```python
from build123d import *

# Parameters (mm, degrees)
SKETCH_1_W       = 100
SKETCH_1_H       = 50
EXTRUDE_1_DEPTH  = 10
F_10_0MM_1_D     = 10
F_10_0MM_1_DEPTH = 23.75
F_10_0MM_1_TIP   = 3.004303095
M10X1_25_1_D     = 8.8
M10X1_25_1_DEPTH = 23.75
M10X1_25_1_TIP   = 2.643786724
FILLET_1_R       = 1
CHAMFER_1_SIZE   = 1
CHAMFER_2_SIZE   = 0.5
FILLET_2_R       = 1


with BuildPart() as part:
    # 草圖1 → 填料-伸長1 (new body)
    with BuildSketch(Plane(origin=(0, 0, 0), x_dir=(1, 0, 0), z_dir=(0, 1, 0))):
        with Locations((50, 25)):
            Rectangle(SKETCH_1_W, SKETCH_1_H)
    extrude(amount=EXTRUDE_1_DEPTH)

    # Ø10.0mm 定位孔1
    with Locations(Plane(origin=(80, 10, -37.5), x_dir=(0, 0, 1), z_dir=(0, 1, 0))):
        with Locations((0, 0), (25, 0)):
            Hole(F_10_0MM_1_D / 2, depth=F_10_0MM_1_DEPTH)
            with Locations((0, 0, -(F_10_0MM_1_DEPTH + F_10_0MM_1_TIP / 2))):  # 118° drill point
                Cone(0, F_10_0MM_1_D / 2, F_10_0MM_1_TIP, mode=Mode.SUBTRACT)

    # M10x1.25 螺紋孔1
    with Locations(Plane(origin=(20, 10, -37.5), x_dir=(0, 0, 1), z_dir=(0, 1, 0))):
        with Locations((0, 0), (25, 0)):
            Hole(M10X1_25_1_D / 2, depth=M10X1_25_1_DEPTH)
            with Locations((0, 0, -(M10X1_25_1_DEPTH + M10X1_25_1_TIP / 2))):  # 118° drill point
                Cone(0, M10X1_25_1_D / 2, M10X1_25_1_TIP, mode=Mode.SUBTRACT)

    # 圓角1
    fillet_1_edges = [part.edges().sort_by_distance(p)[0] for p in [
        (0, 5, -50),
        (100, 5, -50),
        (100, 5, 0),
        (0, 5, 0),
    ]]
    fillet(fillet_1_edges, radius=FILLET_1_R)

    # 導角1
    chamfer_1_edges = [part.edges().sort_by_distance(p)[0] for p in [
        (50, 0, -50),
        (0, 0, -25),
        (100, 0, -25),
        (50, 0, 0),
        (99.707106781, 0, -0.292893219),
        (0.292893219, 0, -0.292893219),
        (0.292893219, 0, -49.707106781),
        (99.707106781, 0, -49.707106781),
    ]]
    chamfer(chamfer_1_edges, length=CHAMFER_1_SIZE)

    # 導角2
    chamfer_2_edges = [part.edges().sort_by_distance(p)[0] for p in [
        (80, 10, -7.5),
        (80, 10, -32.5),
    ]]
    chamfer(chamfer_2_edges, length=CHAMFER_2_SIZE)

    # 圓角2
    fillet_2_edges = [part.edges().sort_by_distance(p)[0] for p in [
        (50, 10, -50),
        (100, 10, -25),
        (0, 10, -25),
        (50, 10, 0),
        (99.707106781, 10, -0.292893219),
        (0.292893219, 10, -0.292893219),
        (0.292893219, 10, -49.707106781),
        (99.707106781, 10, -49.707106781),
    ]]
    fillet(fillet_2_edges, radius=FILLET_2_R)


solid = part.part
```
Check sheet for the modelled part. Datum: model origin and axes. Units: mm. Give positions to 0.01 mm unless a question says otherwise; leave off trailing zeros. Write each loop counter-clockwise with the first axis right and the second up, starting at its lowest first coordinate (ties: lowest second). Pieces come first, ordered by that corner, then holes.
Item 1: Cross-section at A-A (x = 20). Enter the section's corners in (y, z), and give its area (3 significant figures).
Item 2: Cross-section at B-B (z = -37.5). Enter the section's corners in (x, y).
Item 3: Draft check along X on faces 1 (the face through (21.322, 4.93, -41.697)), 2 (the face through (100, 5, -25)), 3 (the face through (49, 5, -50)), 4 (the face through (75.12, 4.68, -11.42)). Enter one of: released by +X, released by -X, zero draft, split by the parting line, or undercut.
Item 4: Cross-section at D-D (x = 80). Enter the section's corners in (y, z).
Item 5: Scan lines: L1, parallel to X at y = 2.25, z = -12.5; L2, parallel to Z at x = 82, y = 5; L3, parallel to Z at x = 76, y = 1.5. Record each from-to range of solid material in increasing order.
Item 6: Cross-section at C-C (y = 8). Enter the section's corners in (x, z), and give its area (3 significant figures).
Report:
1. outline: (0, -49) - (1, -50) - (9, -50) arc R1 ccw to (10, -49) - (10, -41.9) - (0, -41.9) - close; (0, -33.1) - (10, -33.1) - (10, -16.9) - (0, -16.9) - close; (0, -8.1) - (10, -8.1) - (10, -1) arc R1 ccw to (9, 0) - (1, 0) - (0, -1) - close
1. area: 323 mm2
2. outline: (0, 1) - (1, 0) - (15.6, 0) - (15.6, 10) - (1, 10) arc R1 ccw to (0, 9) - close; (24.4, 0) - (75, 0) - (75, 9.5) - (74.5, 10) - (24.4, 10) - close; (85, 0) - (99, 0) - (100, 1) - (100, 9) arc R1 ccw to (99, 10) - (85.5, 10) - (85, 9.5) - close
3. face 1: undercut
3. face 2: released by +X
3. face 3: zero draft
3. face 4: undercut
4. outline: (0, -49) - (1, -50) - (9, -50) arc R1 ccw to (10, -49) - (10, -43) - (9.5, -42.5) - (0, -42.5) - close; (0, -32.5) - (9.5, -32.5) - (10, -32) - (10, -18) - (9.5, -17.5) - (0, -17.5) - close; (0, -7.5) - (9.5, -7.5) - (10, -7) - (10, -1) arc R1 ccw to (9, 0) - (1, 0) - (0, -1) - close
5. L1: x = 0 to 15.6, 24.4 to 75, 85 to 100
5. L2: z = -50 to -42.08, -32.92 to -17.08, -7.92 to 0
5. L3: z = -50 to -40.5, -34.5 to -15.5, -9.5 to 0
6. outline: (0, -49) arc R1 ccw to (1, -50) - (99, -50) arc R1 ccw to (100, -49) - (100, -1) arc R1 ccw to (99, 0) - (1, 0) arc R1 ccw to (0, -1) - close; hole circle Ø8.8 at (20, -37.5); hole circle Ø8.8 at (20, -12.5); hole circle Ø10 at (80, -37.5); hole circle Ø10 at (80, -12.5)
6. area: 4,720 mm2
